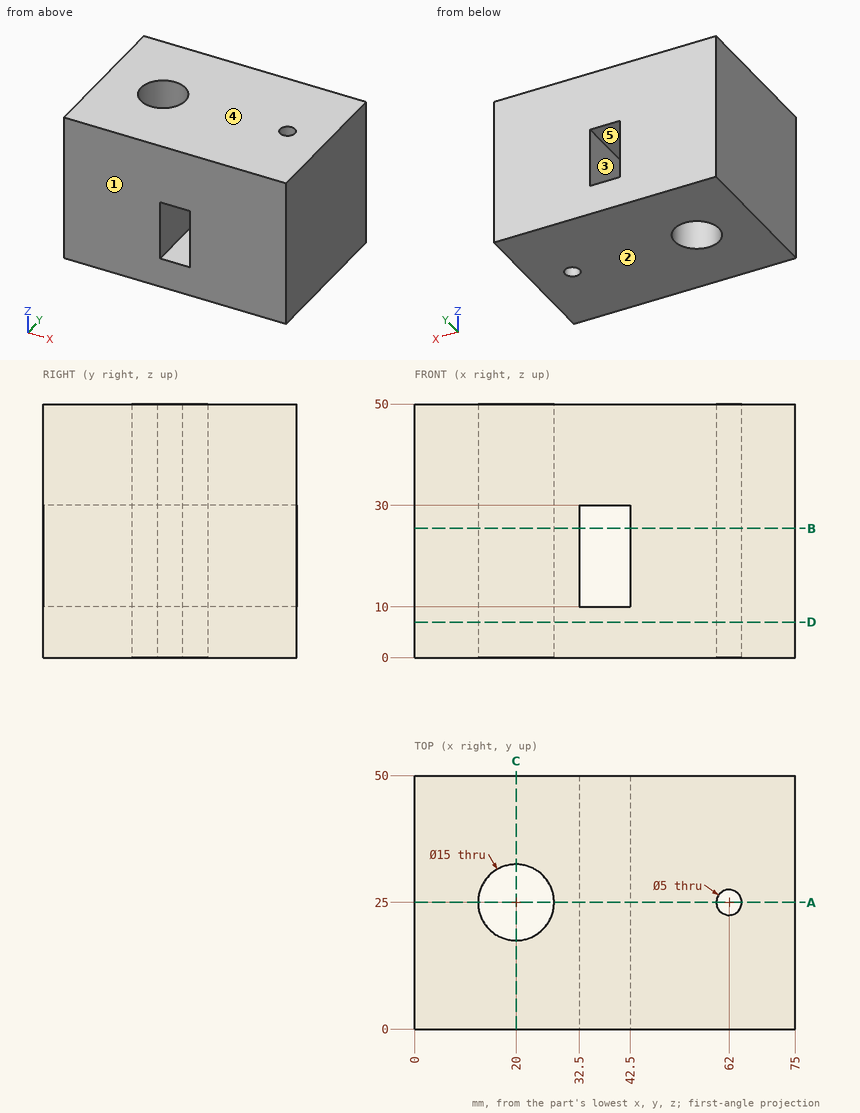
The figure shows three views and two pictorial views of one solid part (mm, origin at its lowest corner). Answer the questions. A direction names the side the tool comes from. Coordinates: 2 decimals unless noted, no trailing zeros. Write each loop counter-clockwise with the first axis right and the second up, starting at its lowest first coordinate (ties: lowest second). Pieces come first, ordered by that corner, then holes. Notation, with made-up numbers: (7.25, -14.75) -> (41.25, -14.75) arc R13 cw to (41.25, -10.75) -> close; hole circle Ø3 at (37, 77.25). An arc over 180 degrees is marked (long way). Return JSON: item names as keys, results as strings.
1. A tool of negligible diameter and unlimited length cuts with its end or side. For the marked faces 4 and 5, from which of +Z, -Z, +X, -X, +Y, -Y can it reach the whole face along a straight path? Write none if from no direction.
Found:
{"face 4": "+Z, +X, -X, +Y, -Y", "face 5": "+Y, -Y"}
2. A cutting plane is placed at D-D (z = 7). Determine the outline of the cut face in (x, y), and give its area (3 significant figures).
Found:
{"outline": "(0, 0) -> (75, 0) -> (75, 50) -> (0, 50) -> close; hole circle Ø15 at (20, 25); hole circle Ø5 at (62, 25)", "area": "3,550 mm2"}
3. A cutting plane is placed at A-A (y = 25). Determine the outline of the cut face in (x, z), and give its area (3 significant figures).
Found:
{"outline": "(0, 0) -> (12.5, 0) -> (12.5, 50) -> (0, 50) -> close; (27.5, 0) -> (59.5, 0) -> (59.5, 50) -> (27.5, 50) -> close; (64.5, 0) -> (75, 0) -> (75, 50) -> (64.5, 50) -> close; hole (32.5, 10) -> (42.5, 10) -> (42.5, 30) -> (32.5, 30) -> close", "area": "2,550 mm2"}
4. Each of these flat-tipped pins is pushed along its axis until it touches: P1, Ø5, axis at x = 38.5, y = 31.5, coming from the -Z side; P2, Ø8, axis at x = 21, y = 24.5, coming from the -Z side. Where does it stop, or does it pass through?
Found:
{"P1": "z = 0", "P2": "through"}
5. A cutting plane is placed at C-C (x = 20). Determine the outline of the cut face in (y, z), and give its area (3 significant figures).
Found:
{"outline": "(0, 0) -> (17.5, 0) -> (17.5, 50) -> (0, 50) -> close; (32.5, 0) -> (50, 0) -> (50, 50) -> (32.5, 50) -> close", "area": "1,750 mm2"}
6. Find the intervals of material crossed by line 1 along X through (y, z) = (35, 19); line 2 along Z through (x, y) = (42, 38); line 3 along Y through (x, z) = (20, 31), in increasing order. Write a range as from..to.
Found:
{"line 1": "0..32.5, 42.5..75", "line 2": "0..10, 30..50", "line 3": "0..17.5, 32.5..50"}
7. Determine the mould class of the marked faces 1, 2 and 3 for opening direction Z: pulls with the +Z half, pulls with the -Z half, needs draft (parallel to the pull), parting line crosses it, or undercut.
Found:
{"face 1": "needs draft", "face 2": "pulls with the -Z half", "face 3": "undercut"}
8. A cutting plane is placed at B-B (z = 25.5). Determine the outline of the cut face in (x, y).
Found:
{"outline": "(0, 0) -> (32.5, 0) -> (32.5, 50) -> (0, 50) -> close; (42.5, 0) -> (75, 0) -> (75, 50) -> (42.5, 50) -> close; hole circle Ø15 at (20, 25); hole circle Ø5 at (62, 25)"}
